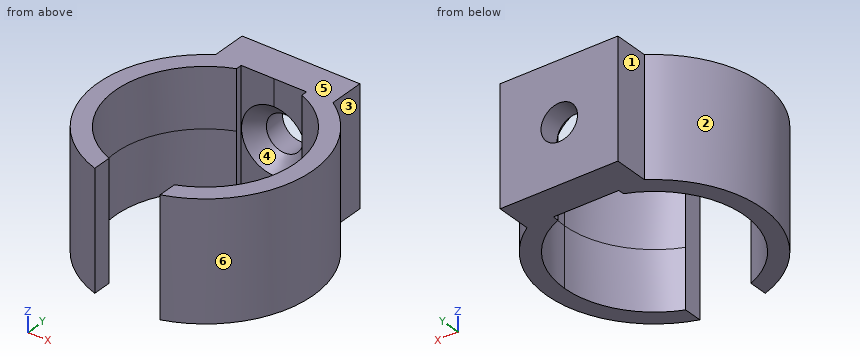
from build123d import *

# Parameters (mm, degrees)
F1_DEPTH       = 5
F1_DEPTH_BACK  = 5
F2_W           = 5.55
F2_H           = 10
F3_DEPTH       = 25
F5_D           = 3.1
F5_CSINK_D     = 5.5
F5_CSINK_ANGLE = 90


with BuildPart() as f1:
    # F0 (on Top) → F1 (new body, two sides)
    with BuildSketch(Plane.XY) as f1_sk:
        with BuildLine():
            Line((5.0199601592, 0), (5.0199601592, 3))
            Line((5.0199601592, 3), (-4.9800398408, 3))
            Line((-4.9800398408, 3), (-4.9800398408, 0.0260473672))
            ThreePointArc((-4.9800398408, 0.0260473672), (0.0238332602, 1.4999689604), (5.0199601592, 0))
        make_face()
        with BuildLine():
            ThreePointArc((9.15, -7.65), (8.0515568512, -3.3031698594), (5.0199601592, 0))
            Line((5.0199601592, 0), (0, 0))
            Line((0, 0), (-4.9800398408, 0))
            Line((-4.9800398408, 0), (-4.9800398408, 0.0260473672))
            ThreePointArc((-4.9800398408, 0.0260473672), (-4.3677875095, -15.6902072282), (9.15, -7.65))
        make_face()
        with BuildLine():
            ThreePointArc((7.65, -7.65), (-5.4093668761, -13.0593668761), (0, 0))
            ThreePointArc((0, 0), (5.4093668761, -2.2406331239), (7.65, -7.65))
        make_face(mode=Mode.SUBTRACT)
        with BuildLine():
            Line((0, 0), (5.0199601592, 0))
            ThreePointArc((5.0199601592, 0), (0.0238332602, 1.4999689604), (-4.9800398408, 0.0260473672))
            Line((-4.9800398408, 0.0260473672), (-4.9800398408, 0))
            Line((-4.9800398408, 0), (0, 0))
        make_face()
    extrude(amount=F1_DEPTH)
    extrude(f1_sk.sketch, amount=-F1_DEPTH_BACK)

    # F2 (on Front) → F3 (cut)
    with BuildSketch(Plane.XZ):
        Rectangle(F2_W, F2_H)
    extrude(amount=F3_DEPTH, mode=Mode.SUBTRACT)

    # F5 (through all)
    with Locations(Plane.XZ):
        with Locations((0, 0)):
            CounterSinkHole(F5_D / 2, F5_CSINK_D / 2, counter_sink_angle=F5_CSINK_ANGLE)


solid = f1.part
CAD build for the part. Positions are in the model's coordinates, mm. Face numbers are marked on the shaded views. A direction names the side the tool comes from. Give positions to 0.01 mm unless a question says otherwise; leave off trailing zeros. Write each loop counter-clockwise with the first axis right and the second up, starting at its lowest first coordinate (ties: lowest second). Pieces come first, ordered by that corner, then holes. Notation, with made-up numbers: M 6,16.5 L 12,16.5 A8 ccw 12,20.5 Z; hole C 51,80 d4. An arc over 180 degrees is marked long. Put each result on its own line as item: value. Start each with the question number.
(1) Band-saw the part on B-B, the plane y = -8.5. Write the cut outline in (x, z), and give its area (3 significant figures).
(2) Which spindle directions (+Z, -Z, +X, -X, +Y, -Y) get a long thin tool onto all of the face, cutting with end or side? Do the marked faces 1, 2 and 3. Say none if no direction does.
(3) Band-saw the part on A-A, the plane x = 5.25. Write the cut outline in (y, z).
(4) Mould opens along Z. For the marked faces 4, 5 and 6 say: +Z half, -Z half, draft (parallel to the pull), parting line (faces both ways), or undercut.
(5) Probe L1, parallel to Z at x = 0, y = 2.15; L2, parallel to X at y = 2.55, z = 0; L3, parallel to Y at x = -3, z = 4.75. List the from-to ranges inside material, lowest first.
(6) Flat gauge pins, fed straight in: pin 1 Ø1.5 at (y, z) = (1, 2) entering from +X; pin 2 Ø0.5 at (y, z) = (-15.5, -0.5) entering from -X; pin 3 Ø0.8 at (y, z) = (-15.5, 0) entering from +X. Where does each tip first touch, or does it go through?
Response values:
1. outline: M -9.11,-5 L -7.6,-5 L -7.6,5 L -9.11,5 Z; M 7.6,-5 L 9.11,-5 L 9.11,5 L 7.6,5 Z
1. area: 30.2 mm2
2. face 1: +Z, -Z, -X, +Y
2. face 2: +Z, -Z, -X
2. face 3: +Z, -Z, +X, +Y
3. outline: M -15.14,-5 L -13.21,-5 L -13.21,5 L -15.14,5 Z; M -2.09,-5 L -0.16,-5 L -0.16,5 L -2.09,5 Z
4. face 4: undercut
4. face 5: +Z half
4. face 6: draft
5. L1: z = -5 to -1.55, 1.55 to 5
5. L2: x = -4.98 to -1.55, 1.55 to 5.02
5. L3: y = -16.29 to -14.69, -0.61 to 3
6. pin 1: stops at x = 5.02
6. pin 2: stops at x = -5.1
6. pin 3: stops at x = 5.31
